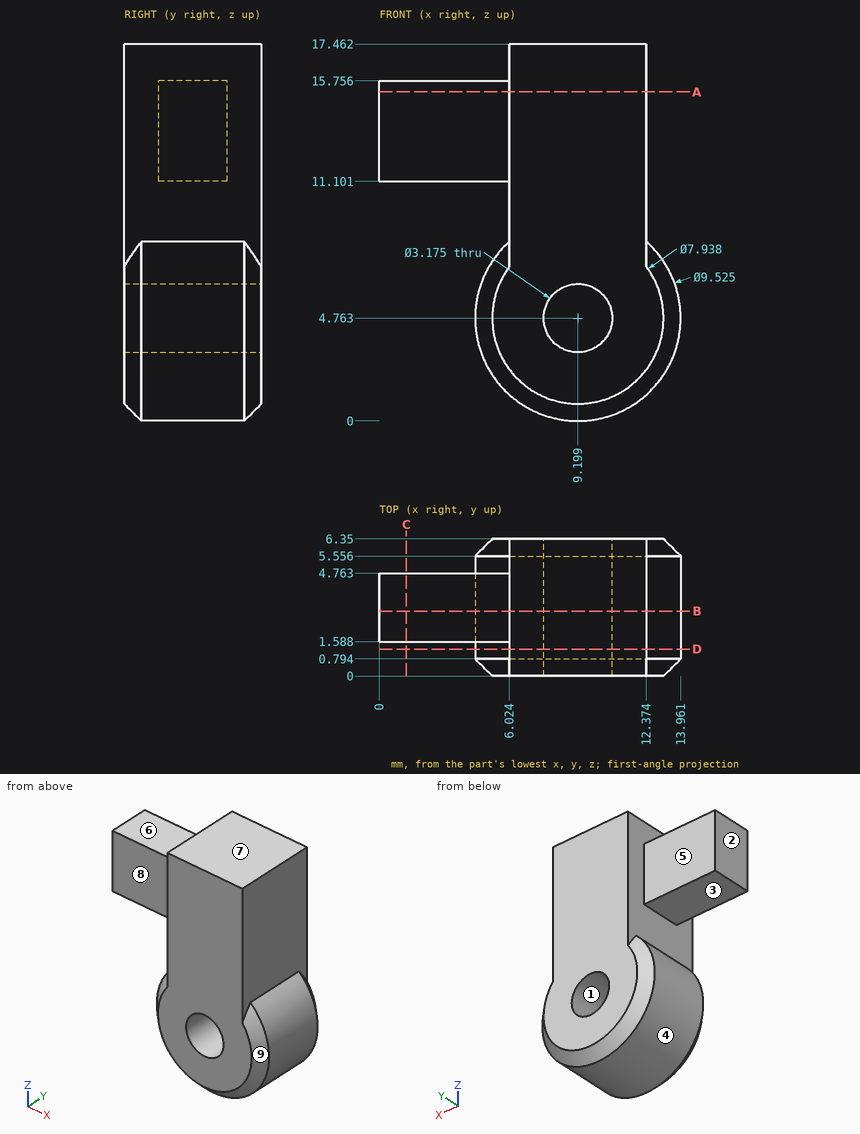
The drawing under review shows one solid part. Ordinate dimensions are in mm from its lowest x, y, z. A direction names the side the tool comes from. Round coordinates to 2 decimals unless told otherwise and drop trailing zeros. Loops run counter-clockwise (first coordinate to the right, second up) from the corner with the lowest first, then second, coordinate; pieces in that order, holes last.
Item 1: Take a section at B-B (y = 3). Write out the cut boundary in (x, z) (1 decimal).
Determined:
outline: (0, 11.1) - (6, 11.1) - (6, 8.3) arc R4.8 ccw (long way) to (12.4, 8.3) - (12.4, 17.5) - (6, 17.5) - (6, 15.8) - (0, 15.8) - close; hole circle Ø3.2 at (9.2, 4.8)
Item 2: Take a section at A-A (z = 15.25). Write out the cut boundary in (x, y).
Determined:
outline: (0, 1.59) - (6.02, 1.59) - (6.02, 0) - (12.37, 0) - (12.37, 6.35) - (6.02, 6.35) - (6.02, 4.76) - (0, 4.76) - close
Item 3: Clearance check with flat-ended pins moving along their axes: pin 1 Ø3.5 at (x, z) = (4, 14) entering from -Y; pin 2 Ø3.5 at (x, y) = (2.5, 3) entering from +Z; pin 3 Ø1.5 at (x, y) = (11.5, 4.5) entering from -Z. State where each tip first meets the part, or that it passes through.
Determined:
pin 1: stops at y = 1.59
pin 2: stops at z = 15.76
pin 3: stops at z = 0.26
Item 4: Take a section at D-D (y = 1.25). Write out the cut boundary in (x, z) (1 decimal), then the cut area to 3 significant figures.
Determined:
outline: (6, 8.3) arc R4.8 ccw (long way) to (12.4, 8.3) - (12.4, 17.5) - (6, 17.5) - close; hole circle Ø3.2 at (9.2, 4.8)
area: 116 mm2
Item 5: Take a section at C-C (x = 1.25). Write out the cut boundary in (y, z) (1 decimal).
Determined:
outline: (1.6, 11.1) - (4.8, 11.1) - (4.8, 15.8) - (1.6, 15.8) - close
Item 6: For line 1 (X direction, y = 3.5, z = 15.5); line 2 (X direction, y = 2.25, z = 9.5); line 3 (Z direction, x = 8.75, y = 2) (1 decimal), list the stretches that pass through material, from the lowest coordinate up.
Determined:
line 1: x = 0 to 12.37
line 2: x = 6.02 to 12.37
line 3: z = 0 to 3.2, 6.3 to 17.5
Item 7: For the marked faces 5, 6, 7, 8 and 9, list the 3-axis set-ups (+Z, -Z, +X, -X, +Y, -Y) from which the entire face can be reached by the end or side of a thin tool; tool diameter is ignored.
Determined:
face 5: +Z, -X, +Y
face 6: +Z, -X, +Y, -Y
face 7: +Z, +X, -X, +Y, -Y
face 8: +Z, -X, -Y
face 9: -Y
Item 8: Mouldability with a two-part tool opening along X and no side actions: class the marked faces 1, 2, 3 and 4 as released by +X, released by -X, zero draft, split by the parting line, or undercut.
Determined:
face 1: undercut
face 2: released by -X
face 3: zero draft
face 4: split by the parting line
